Check sheet for the modelled part. Datum: model origin and axes. Units: mm. A direction names the side the tool comes from. Round coordinates to 2 decimals unless told otherwise and drop trailing zeros. Loops run counter-clockwise (first coordinate to the right, second up) from the corner with the lowest first, then second, coordinate; pieces in that order, holes last. Notation, with made-up numbers: (-18.75, 75) - (18.25, 75) arc R37 ccw to (18.25, 111) - close; hole circle Ø4 at (-17.75, -24). An arc over 180 degrees is marked (long way). Return JSON: item names as keys, results as strings.
from build123d import *

# Parameters (mm, degrees)
SKETCH2_R           = 2
BOSS_EXTRUDE1_DEPTH = 3.5
SHELL1_T            = -0.4


with BuildPart() as part:
    # Sketch1 → Revolve1 (revolve)
    with BuildSketch(Plane.XY):
        with BuildLine():
            Line((0, -2.875), (0, 2.875))
            ThreePointArc((0, 2.875), (-2.875, 0), (0, -2.875))
        make_face()
    revolve(axis=Axis((0, 55, 0), (0, -1, 0)))

    # Sketch2 → Boss-Extrude1 (add, symmetric)
    with BuildSketch(Plane(origin=(0, 0, 0), x_dir=(1, 0, 0), z_dir=(0, 1, 0))):
        Circle(SKETCH2_R)
    extrude(amount=BOSS_EXTRUDE1_DEPTH, both=True)

    # Shell1
    shell1_openings = [part.faces().sort_by_distance(p)[0] for p in [
        (0, 3.5, 0),
        (0, -3.5, 0),
    ]]
    offset(amount=SHELL1_T, openings=shell1_openings, kind=Kind.INTERSECTION)


solid = part.part
Q1. Sectioned sample at C-C (z = -1.7). Enter the section's corners in (x, y), plus the area to 3 significant figures.
Answer key:
{"outline": "(-1.05, -3.5) - (1.05, -3.5) - (1.05, -2.07) arc R2.32 ccw to (1.05, 2.07) - (1.05, 3.5) - (-1.05, 3.5) - (-1.05, 2.07) arc R2.32 ccw to (-1.05, -2.07) - close; hole circle Ø3.6 at (0, 0)", "area": "12.0 mm²"}
Q2. Sectioned sample at B-B (z = 0). Enter the section's corners in (x, y) (3 decimals), plus the area to 3 significant figures.
Answer key:
{"outline": "(-2, -3.5) - (-1.6, -3.5) - (-1.6, -1.888) arc R2.475 cw to (-1.6, 1.888) - (-1.6, 3.5) - (-2, 3.5) - (-2, 2.065) arc R2.875 ccw to (-2, -2.065) - close; (1.6, -3.5) - (2, -3.5) - (2, -2.065) arc R2.875 ccw to (2, 2.065) - (2, 3.5) - (1.6, 3.5) - (1.6, 1.888) arc R2.475 cw to (1.6, -1.888) - close", "area": "6.00 mm²"}
Q3. Tool access check on faces 3 (the face through (-1.27, -2.68, 0.97)), 4 (the face through (0, -3, 2)). Record the directions out of +Z, -Z, +X, -X, +Y, -Y that give a thin tool (end or side, any length) a straight path to the whole face; none if there is none.
Answer key:
{"face 3": "+Y, -Y", "face 4": "-Y"}
Q4. Draft check along Z on faces 1 (the face through (-1.27, 2.71, 0.97)), 2 (the face through (0, 3, 2)). Enter one of: released by +Z, released by -Z, zero draft, split by the parting line, or undercut.
Answer key:
{"face 1": "undercut", "face 2": "split by the parting line"}
Q5. Scan lines: probe 1 along Z at (x, y) = (0, -2.5); probe 2 along Z at (x, y) = (-0.9, -1.75); probe 3 along X at (y, z) = (2.5, -0.2). Record each from-to range of solid material in increasing order. Write a range as [from, to].
Answer key:
{"probe 1": "z = [-2, -1.6], [1.6, 2]", "probe 2": "z = [-2.1, -1.5], [1.5, 2.1]", "probe 3": "x = [-1.99, -1.59], [1.59, 1.99]"}
Q6. Sectioned sample at A-A (x = 0). Enter the section's corners in (y, z) (3 decimals).
Answer key:
{"outline": "(-3.5, -2) - (-2.065, -2) arc R2.875 ccw to (2.065, -2) - (3.5, -2) - (3.5, -1.6) - (1.888, -1.6) arc R2.475 cw to (-1.888, -1.6) - (-3.5, -1.6) - close; (-3.5, 1.6) - (-1.888, 1.6) arc R2.475 cw to (1.888, 1.6) - (3.5, 1.6) - (3.5, 2) - (2.065, 2) arc R2.875 ccw to (-2.065, 2) - (-3.5, 2) - close"}
Q7. Depth check by flat-ended pin: P1, Ø2.5, axis at x = 0, z = 0, coming from the +Y side; P2, Ø3, axis at y = 1, z = 1.5, coming from the +X side; P3, Ø3, axis at y = -2, z = 2, coming from the +X side. Enter the tip coordinate at first touch or a pass-through.
Answer key:
{"P1": "passes through", "P2": "stops at x = 2.86", "P3": "stops at x = 2.55"}
Q8. Sectioned sample at D-D (y = -1.5). Enter the section's corners in (x, z), plus the area to 3 significant figures.
Answer key:
{"outline": "circle Ø4.91 at (0, 0); hole circle Ø3.94 at (0, 0)", "area": "6.72 mm²"}
